from build123d import *

# Parameters (mm, degrees)
CROQUIS1_R              = 1.5
SALIENTE_EXTRUIR1_DEPTH = 2
REDONDEO1_R             = 1


with BuildPart() as part:
    # Croquis1 → Saliente-Extruir1 (new body)
    with BuildSketch(Plane.XY):
        with BuildLine():
            Line((15, 3.5), (-15, 3.5))
            ThreePointArc((-15, 3.5), (-21.031506006, 6.945719569), (-20.936491673, 0))
            Line((-20.936491673, 0), (20.936491673, 0))
            ThreePointArc((20.936491673, 0), (21.031506006, 6.945719569), (15, 3.5))
        make_face()
        with Locations((-19, 3.5)):
            Circle(CROQUIS1_R, mode=Mode.SUBTRACT)
        with Locations((19, 3.5)):
            Circle(CROQUIS1_R, mode=Mode.SUBTRACT)
    extrude(amount=SALIENTE_EXTRUIR1_DEPTH)

    # Redondeo1
    redondeo1_edges = [part.edges().sort_by_distance(p)[0] for p in [
        (20.936491673, 0, 1),
        (-20.936491673, 0, 1),
        (-15, 3.5, 1),
        (15, 3.5, 1),
    ]]
    fillet(redondeo1_edges, radius=REDONDEO1_R)


solid = part.part
Source: CAD feature listing. Evaluate the final solid. Frame: model axes, mm. A direction names the side the tool comes from. Coordinates: 2 decimals unless noted, no trailing zeros. Loops run counter-clockwise (first coordinate to the right, second up) from the corner with the lowest first, then second, coordinate; pieces in that order, holes last. Notation, with made-up numbers: (-15, 40.5) - (37, 40.5) arc R19 cw to (37, 77.5) - close; hole circle Ø11 at (-7.5, -10.75). An arc over 180 degrees is marked (long way). Return JSON: item names as keys, results as strings.
Q1. Section D-D, the plane x = -15.5. Return loops of the section in (y, z).
Results:
{"outline": "(0, 0) - (5.44, 0) - (5.44, 2) - (0, 2) - close"}
Q2. Section A-A, the plane x = 19. Return loops of the section in (y, z), plus the area to 3 significant figures.
Results:
{"outline": "(0, 0) - (2, 0) - (2, 2) - (0, 2) - close; (5, 0) - (7.5, 0) - (7.5, 2) - (5, 2) - close", "area": "9.00 mm2"}
Q3. Section C-C, the plane x = -10.5. Return loops of the section in (y, z), plus the area to 3 significant figures.
Results:
{"outline": "(0, 0) - (3.5, 0) - (3.5, 2) - (0, 2) - close", "area": "7.00 mm2"}
Q4. Material intervals for line 1 along Y through (x, z) = (19, 1.2); line 2 along X through (y, z) = (4, 1.3); line 3 along X through (y, z) = (3, 1.8), sorted ascending.
Results:
{"line 1": "0 to 2, 5 to 7.5", "line 2": "-22.97 to -20.41, -17.59 to -14.97, 14.97 to 17.59, 20.41 to 22.97", "line 3": "-22.97 to -20.41, -17.59 to 17.59, 20.41 to 22.97"}
Q5. Contact query for a flat-ended pin moving along its axis: P1, Ø1, axis at x = -4, z = 1, coming from the +Y side. Output: stop coordinate, or through.
Results:
{"P1": "y = 3.5"}
Q6. Section B-B, the plane z = 1.15. Return loops of the section in (x, y), plus the area to 3 significant figures.
Results:
{"outline": "(-21.21, 0.17) arc R1 ccw to (-20.66, 0) - (20.66, 0) arc R1 ccw to (21.21, 0.17) arc R4 ccw (long way) to (15.08, 4.3) arc R1 cw to (14.1, 3.5) - (-14.1, 3.5) arc R1 cw to (-15.08, 4.3) arc R4 ccw (long way) to start; hole circle Ø3 at (-19, 3.5); hole circle Ø3 at (19, 3.5)", "area": "193 mm2"}
Q7. Access query for faces 1 (the cylindrical face through (17.5, 3.57, 0.99)), 2 (the cylindrical face through (14.7, 3.7, 1)). Directions: +Z, -Z, +X, -X, +Y, -Y. A direction counts if a zero-diameter tool reaches every point of the face in a straight line with its end or side. Return the directions, or none.
Results:
{"face 1": "+Z, -Z", "face 2": "+Z, -Z, +Y"}
Q8. Mould query, pull axis Y, two halves, no side actions, for faces 3 (the flat face through (0, 0, 1)), 4 (the cylindrical face through (-20.5, 3.57, 0.99)), 5 (the flat face through (0, 3, 0)). Classes: released by +Y, released by -Y, zero draft, split by the parting line, or undercut.
Results:
{"face 3": "released by -Y", "face 4": "undercut", "face 5": "zero draft"}
